Design review of the part built by this model. Coordinates are the model's own, in mm. A direction names the side the tool comes from. Coordinates: 2 decimals unless noted, no trailing zeros. Loops run counter-clockwise (first coordinate to the right, second up) from the corner with the lowest first, then second, coordinate; pieces in that order, holes last. Notation, with made-up numbers: (74, 74.5) - (93, 74.5) arc R22 cw to (93, 86.5) - close; hole circle Ø1 at (-30.5, 71). An arc over 180 degrees is marked (long way). Answer in a Markdown table with one row per item. Add a question column.
(1) Clearance check with flat-ended pins moving along their axes: pin 1 (5 mm diameter, centred on y = -60, z = 58.5, fed in from -X); pin 2 (3 mm diameter, centred on y = 31.5, z = 56, fed in from +X); pin 3 (3.5 mm diameter, centred on x = -24, y = -48, fed in from -Z). State where each tip first meets the part, or that it passes through.
(2) To check wall thickness, follow L1, parallel to X at y = -50, z = 76; L2, parallel to Z at x = -18, y = -9.5; L3, parallel to X at y = -5, z = 17. State the ranges of each line that lie inside material, in increasing order. Write a range as [from, to].
(3) For faces 1 (the face through (-23, -43, 3)), 2 (the face through (-22, 1, 0)), 3 (the face through (-23, 30, 3)), 4 (the face through (-16, 1, 3)), list the 3-axis set-ups (+Z, -Z, +X, -X, +Y, -Y) from which the entire face can be reached by the end or side of a thin tool; tool diameter is ignored.
(4) We need section C-C, the plane x = -15. Write out the cut boundary in (y, z), plus the area to 3 significant figures.
(5) We need section B-B, the plane z = 16. Write out the cut boundary in (x, y), plus the area to 3 significant figures.
(6) We need section A-A, the plane y = 5.5. Write out the cut boundary in (x, z).
(7) We need section D-D, the plane z = 29.5. Write out the cut boundary in (x, y).
from build123d import *

# Parameters (mm, degrees)
SKETCH_2_W      = 23.702391565
SKETCH_2_H      = 23.489524234
EXTRUDE_1_DEPTH = 3
SKETCH_3_W      = 3.165508912
SKETCH_3_H      = 123.567997976
EXTRUDE_2_DEPTH = 100
FILLET_1_R      = 30


with BuildPart() as part:
    # 草图2 → 凸台-拉伸1 (new body)
    with BuildSketch(Plane.XY):
        with Locations((-21.737891338, 0.42425972)):
            Rectangle(SKETCH_2_W, SKETCH_2_H)
    extrude(amount=EXTRUDE_1_DEPTH)

    # 草图3 → 凸台-拉伸2 (add)
    with BuildSketch(Plane.XY.offset(3)):
        with Locations((-23.40524573, -14.022020715)):
            Rectangle(SKETCH_3_W, SKETCH_3_H)
    extrude(amount=EXTRUDE_2_DEPTH)

    # 圆角1
    # the kernel refuses this fillet: 30 mm, written as the material it adds along each edge
    with BuildSketch(Plane(origin=(-24.988000186, 12.169021837, 3), x_dir=(-1, 0, 0), z_dir=(0, -1, 0))) as fillet_1_piece_1:
        with BuildLine():
            CenterArc((30, -21.025853601), FILLET_1_R, 135.503813775, 44.496186225)
            Line((0, -21.025853601), (0, 0))
            Line((0, 0), (8.601086935, 0))
        make_face()
    extrude(amount=23.489524234)


solid = part.part
Responses:
| question | item | result |
|---|---|---|
| 1 | pin 1 | stops at x = -24.99 |
| 1 | pin 2 | stops at x = -21.82 |
| 1 | pin 3 | stops at z = 3 |
| 2 | L1 | x = [-24.99, -21.82] |
| 2 | L2 | z = [0, 3] |
| 2 | L3 | x = [-25.82, -21.82] |
| 3 | face 1 | -Z, +X, -X, -Y |
| 3 | face 2 | -Z, +X, -X, +Y, -Y |
| 3 | face 3 | -Z, +X, -X, +Y |
| 3 | face 4 | +Z, +X, +Y, -Y |
| 4 | outline | (-11.32, 0) - (12.17, 0) - (12.17, 3) - (-11.32, 3) - close |
| 4 | area | 70.5 mm2 |
| 5 | outline | (-26.08, -11.32) - (-24.99, -11.32) - (-24.99, -75.81) - (-21.82, -75.81) - (-21.82, 47.76) - (-24.99, 47.76) - (-24.99, 12.17) - (-26.08, 12.17) - close |
| 5 | area | 417 mm2 |
| 6 | outline | (-33.59, 0) - (-9.89, 0) - (-9.89, 3) - (-21.82, 3) - (-21.82, 103) - (-24.99, 103) - (-24.99, 24.03) arc R30 cw to (-33.59, 3) - close |
| 7 | outline | (-24.99, -75.81) - (-21.82, -75.81) - (-21.82, 47.76) - (-24.99, 47.76) - close |
